Verification items for the finished model (mm, model axes). Face numbers are marked on the shaded views. Coordinates: 2 decimals unless noted, no trailing zeros. Write each loop counter-clockwise with the first axis right and the second up, starting at its lowest first coordinate (ties: lowest second). Pieces come first, ordered by that corner, then holes. Notation, with made-up numbers: (64, 63.25) -> (82, 63.25) arc R33 cw to (82, 91.25) -> close; hole circle Ø8 at (66, -30.5). An arc over 180 degrees is marked (long way). Use CSV: the item, a comma, the result in double quotes.
```python
from build123d import *

# Parameters (mm, degrees)
SKETCH1_W           = 132
SKETCH1_H           = 132
BOSS_EXTRUDE1_DEPTH = 9
SHELL1_T            = 2
SKETCH2_W           = 175.70161203
SKETCH2_H           = 38.948555966
CUT_EXTRUDE1_DEPTH  = 2
FILLET1_R           = 1
FILLET2_R           = 3
BOSS_EXTRUDE2_START = -2
BOSS_EXTRUDE2_DEPTH = 2
FILLET3_R           = 3


with BuildPart() as part:
    # Sketch1 → Boss-Extrude1 (new body)
    with BuildSketch(Plane(origin=(0, 0, 0), x_dir=(1, 0, 0), z_dir=(0, 1, 0))):
        Rectangle(SKETCH1_W, SKETCH1_H)
    extrude(amount=BOSS_EXTRUDE1_DEPTH)

    # Shell1
    shell1_openings = [part.faces().sort_by_distance(p)[0] for p in [
        (0, 9, 0),
    ]]
    offset(amount=SHELL1_T, openings=shell1_openings, kind=Kind.INTERSECTION)

    # Sketch2 → Cut-Extrude1 (cut)
    with BuildSketch(Plane.ZY.offset(68)):
        Rectangle(SKETCH2_W, SKETCH2_H)
    extrude(amount=-CUT_EXTRUDE1_DEPTH, mode=Mode.SUBTRACT)

    # Fillet1
    fillet1_edges = [part.edges().sort_by_distance(p)[0] for p in [
        (0, 0, 66),
        (66, 0, 0),
        (66, 4.5, 66),
        (0, 0, -66),
        (66, 4.5, -66),
    ]]
    fillet(fillet1_edges, radius=FILLET1_R)

    # Fillet2
    fillet2_edges = [part.edges().sort_by_distance(p)[0] for p in [
        (1, -2, 68),
        (1, -2, -68),
        (68, -2, 0),
        (68, 3.5, -68),
        (68, 3.5, 68),
    ]]
    fillet(fillet2_edges, radius=FILLET2_R)

    # Sketch4 → Boss-Extrude2 (add)
    with BuildSketch(Plane(origin=(0, 9, 0), x_dir=(1, 0, 0), z_dir=(0, 1, 0)).offset(BOSS_EXTRUDE2_START)):
        with BuildLine():
            Line((-66, 82), (-66, 68))
            Line((-66, 68), (65, 68))
            ThreePointArc((65, 68), (67.121320344, 67.121320344), (68, 65))
            Line((68, 65), (68, -65))
            ThreePointArc((68, -65), (67.121320344, -67.121320344), (65, -68))
            Line((65, -68), (-66, -68))
            Line((-66, -68), (-66, -82))
            Line((-66, -82), (65, -82))
            ThreePointArc((65, -82), (77.02081528, -77.02081528), (82, -65))
            Line((82, -65), (82, 65))
            ThreePointArc((82, 65), (77.02081528, 77.02081528), (65, 82))
            Line((65, 82), (-66, 82))
        make_face()
    extrude(amount=BOSS_EXTRUDE2_DEPTH)

    # Fillet3
    fillet3_edges = [part.edges().sort_by_distance(p)[0] for p in [
        (-0.5, 7, 68),
        (67.121320344, 7, 67.121320344),
        (68, 7, 0),
        (67.121320344, 7, -67.121320344),
        (-0.5, 7, -68),
    ]]
    fillet(fillet3_edges, radius=FILLET3_R)


solid = part.part
```
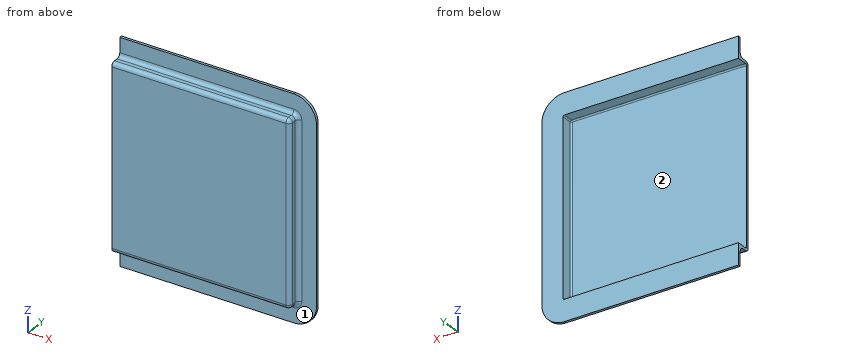
1) Scan lines: L1, parallel to Z at x = 25, y = 7.5; L2, parallel to Y at x = -31.5, z = -28; L3, parallel to Z at x = -22, y = 0.75. Record each from-to range of solid material in increasing order.
Return value:
L1,"-82 to -66, 66 to 82"
L2,"-2 to 0"
L3,"-67.99 to -65.97, 65.97 to 67.99"
2) Mould release check, pull along Z, two halves, no side actions. Record for the marked faces 1 and 2: released by +Z, released by -Z, zero draft, split by the parting line, or undercut.
Return value:
face 1,"zero draft"
face 2,"undercut"
3) Cross-section at B-B (z = 28). Record the boundary of the cut face in (x, y).
Return value:
outline,"(-66, -2) -> (65, -2) arc R3 ccw to (68, 1) -> (68, 4) arc R3 cw to (71, 7) -> (82, 7) -> (82, 9) -> (66, 9) -> (66, 1) arc R1 cw to (65, 0) -> (-66, 0) -> close"
4) Gauge pin test, flat ends, axial feed: pin 1 (3 mm diameter, centred on x = -39.5, y = 0.5, fed in from +Z); pin 2 (4 mm diameter, centred on x = 5, y = 4, fed in from -Z); pin 3 (6.5 mm diameter, centred on x = -1.5, y = 4, fed in from +Z); pin 4 (3.5 mm diameter, centred on x = -18.5, y = 2.5, fed in from -Z). Record the tip position at first contact, or that the pin passes through.
Return value:
pin 1,"z = 68"
pin 2,"z = -68.76"
pin 3,"z = 82"
pin 4,"z = -68.01"
5) Cross-section at A-A (x = -12.5). Record the boundary of the cut face in (y, z), plus the area to 3 significant figures.
Return value:
outline,"(-2, -65) arc R3 ccw to (1, -68) -> (4, -68) arc R3 cw to (7, -71) -> (7, -82) -> (9, -82) -> (9, -66) -> (1, -66) arc R1 cw to (0, -65) -> (0, 65) arc R1 cw to (1, 66) -> (9, 66) -> (9, 82) -> (7, 82) -> (7, 71) arc R3 cw to (4, 68) -> (1, 68) arc R3 ccw to (-2, 65) -> close"
area,"364 mm2"
